The listing builds one solid part. Answer for the finished solid, in the listing's coordinates (mm). A direction names the side the tool comes from. Coordinates: 2 decimals unless noted, no trailing zeros. Order: outer loops, then holes, each group sorted by start corner. A loop starts at its lowest first (then second) coordinate and runs counter-clockwise, first axis right, second up. Notation, with made-up numbers: (-2, 48.5) - (6, 48.5) arc R14 cw to (6, 62.5) - close; hole circle Ø9 at (52.25, 17.25). An arc over 180 degrees is marked (long way). Use one line per item in the form item = value. Start each with the question number.
Item 1: Consider line 1 along Y through (x, z) = (-219.5, 60.5); line 2 along Z through (x, y) = (-213.5, -413); line 3 along Y through (x, z) = (-226, 36.5). Determine where each line is inside the solid, lowest interval first. Write a range as [from, to].
Item 2: A tool of negligible diameter and unlimited length cuts with its end or side. For faces 4 (the flat face through (-219, -211, 60.325)), 5 (the flat face through (-209.039, -202, 37)), 6 (the flat face through (-221.739, -2, 40.3)), from which of +Z, -Z, +X, -X, +Y, -Y can it reach the whole face along a straight path? Write none if from no direction.
Item 3: The mould has two halves that part along Y. Classify faces 1 (the flat face through (-219, 0, 79)), 2 (the flat face through (-219, -212, 0)), 3 (the cylindrical face through (-224.96, -4.52, 32.54)): released by +Y, released by -Y, zero draft, split by the parting line, or undercut.
Item 4: Section C-C, the plane z = 75.5 is taken. Write down the section's boundary in (x, y).
Item 5: Section A-A, the plane x = -214.5 is taken. Write down the section's boundary in (y, z) (3 decimals).
Item 6: Section B-B, the plane y = -162 is taken. Write down the section's boundary in (x, z) (3 decimals).
Item 7: Each of these flat-tipped pins is pushed along its axis until it touches: pin 1 Ø1.6 at (x, y) = (-222, -450) entering from +Z (3 decimals); pin 2 Ø9.5 at (x, y) = (-218, -263) entering from +Z (3 decimals); pin 3 Ø2 at (x, z) = (-217, 14.5) entering from +Y. Where does it stop, or does it pass through?
from build123d import *

# Parameters (mm, degrees)
SKETCH1_W                                        = 19.05
SKETCH1_H                                        = 450.85
BOSS_EXTRUDE1_DEPTH                              = 66.675
FILLET4_R                                        = 38.1
CUT_EXTRUDE1_REACH                               = 458.151
BOSS_EXTRUDE2_DEPTH                              = 19.05
BOSS_EXTRUDE3_DEPTH                              = 19.05
F_1_4_0_25_DIAMETER_HOLE1_D                      = 6.35
F_10_CLEARANCE_HOLE_WITH_1_0_X_25_CB_D           = 5.6134
F_10_CLEARANCE_HOLE_WITH_1_0_X_25_CB_CBORE_D     = 12.7
F_10_CLEARANCE_HOLE_WITH_1_0_X_25_CB_CBORE_DEPTH = 6.35


with BuildPart() as part:
    # Sketch1 → Boss-Extrude1 (new body)
    with BuildSketch(Plane.XY):
        with Locations((-218.563766336, -225.425)):
            Rectangle(SKETCH1_W, SKETCH1_H)
    extrude(amount=BOSS_EXTRUDE1_DEPTH)

    # Fillet4
    fillet4_edges = [part.edges().sort_by_distance(p)[0] for p in [
        (-218.563766336, -450.85, 66.675),
    ]]
    fillet(fillet4_edges, radius=FILLET4_R)

    # Sketch4 → Cut-Extrude1 (cut, up to next)
    with BuildSketch(Plane.ZY.offset(228.088766336), mode=Mode.PRIVATE) as cut_extrude1_sk1:
        with BuildLine():
            Line((66.675, 0), (66.675, -412.75))
            ThreePointArc((66.675, -412.75), (55.515768363, -439.690768363), (28.575, -450.85))
            Line((28.575, -450.85), (28.575, -444.5))
            ThreePointArc((28.575, -444.5), (51.025640303, -435.200640303), (60.325, -412.75))
            Line((60.325, -412.75), (60.325, 0))
            Line((60.325, 0), (66.675, 0))
        make_face()
    cut_extrude1_tool1 = extrude(cut_extrude1_sk1.sketch, amount=-CUT_EXTRUDE1_REACH, mode=Mode.PRIVATE) & part.part
    add(cut_extrude1_tool1.solids().sort_by_distance((-228.088766, -233.202612, 62.01827))[0], mode=Mode.SUBTRACT)

    # Sketch7 → Boss-Extrude2 (add, through all)
    with BuildSketch(Plane.ZY.offset(228.088766336)):
        Polygon((0, 0), (60.325, 0), (60.325, 34.844553242), (0, 20.824633003), align=None)
    extrude(amount=-BOSS_EXTRUDE2_DEPTH)

    # Sketch8 → Boss-Extrude3 (add, through all)
    with BuildSketch(Plane.ZY.offset(228.088766336)):
        Polygon((60.325, 34.844553242), (83.828599938, 40.306941911), (93.196193981, 0), (60.325, 0), align=None)
    extrude(amount=-BOSS_EXTRUDE3_DEPTH)

    # 1/4 (0.25) Diameter Hole1 (through all)
    with Locations(Plane.ZY.offset(228.088766336)):
        with Locations((28.575, -444.5), (60.325, 0)):
            Hole(F_1_4_0_25_DIAMETER_HOLE1_D / 2)

    # #10 Clearance Hole with 1.0 x .25 CB (through all)
    with Locations(Plane.ZY.offset(228.088766336)):
        with Locations((37.58012522, -0.660555349)):
            CounterBoreHole(F_10_CLEARANCE_HOLE_WITH_1_0_X_25_CB_D / 2, F_10_CLEARANCE_HOLE_WITH_1_0_X_25_CB_CBORE_D / 2, F_10_CLEARANCE_HOLE_WITH_1_0_X_25_CB_CBORE_DEPTH)


solid = part.part
Response:
q1.line_1 = [3.17, 34.89]
q1.line_2 = [0, 60.32]
q1.line_3 = [-443.5, -6.92], [5.6, 29.31]
q2.face_4 = +Z, +X, -X, -Y
q2.face_5 = +Z, -Z, +X, +Y, -Y
q2.face_6 = -X
q3.face_1 = released by -Y
q3.face_2 = zero draft
q3.face_3 = undercut
q4.outline = (-228.09, 0) - (-209.04, 0) - (-209.04, 38.37) - (-228.09, 38.37) - close
q5.outline = (-450.85, 0) - (20.825, 0) - (40.307, 83.829) - (0, 93.196) - (0, 63.5) arc R3.175 cw (long way) to (-3.175, 60.325) - (-412.75, 60.325) arc R31.75 ccw to (-444.341, 31.746) arc R3.175 cw (long way) to (-447.675, 28.575) - (-450.85, 28.575) - close; hole circle Ø5.613 at (-0.661, 37.58)
q6.outline = (-228.089, 0) - (-209.039, 0) - (-209.039, 60.325) - (-228.089, 60.325) - close
q7.pin_1 = 28.575
q7.pin_2 = 60.325
q7.pin_3 = 24.43
